Geometry check sheet. Reference: the model listing, model coordinates, mm. Give positions to 0.01 mm unless a question says otherwise; leave off trailing zeros. Write each loop counter-clockwise with the first axis right and the second up, starting at its lowest first coordinate (ties: lowest second). Pieces come first, ordered by that corner, then holes. Notation, with made-up numbers: M -9.5,-12.5 L 30.5,-12.5 A22 ccw 30.5,23.5 Z; hole C 86,77.5 d6. An arc over 180 degrees is marked long. One line per item, written item: value. Start each with the question number.
1. Cross-section at A-A on x = 38.6. Record the cut outline in (y, z), then the cut area to 3 significant figures.
2. Scan lines: line 1 (X direction, y = -7, z = 0); line 2 (Y direction, x = 5, z = 7); line 3 (Y direction, x = 146.5, z = 0.5). Record each from-to range of solid material in increasing order.
3. Gauge pin test, flat end, axial feed: pin 1 (2.5 mm diameter, centred on x = 170, y = 0, fed in from -Z). Record the tip position at first contact, or that the pin passes through.
4. Cross-section at B-B on x = 135. Record the cut outline in (y, z).
from build123d import *

# Parameters (mm, degrees)
SKETCH_1_W          = 15
SKETCH_1_H          = 15
SKETCH_1_W_2        = 13
SKETCH_1_H_2        = 13
EXTRUDE_1_DEPTH     = 185
SKETCH_2_R          = 1.45
CUT_EXTRUDE_1_DEPTH = 186.758579883
SKETCH_3_R          = 1.6
SKETCH_3_R_2        = 1.45
CUT_EXTRUDE_2_DEPTH = 186.758579883


with BuildPart() as part:
    # 草图1 → 凸台-拉伸1 (new body)
    with BuildSketch(Plane(origin=(0, 0, 0), x_dir=(0, 0, -1), z_dir=(1, 0, 0))):
        Rectangle(SKETCH_1_W, SKETCH_1_H)
        Rectangle(SKETCH_1_W_2, SKETCH_1_H_2, mode=Mode.SUBTRACT)
    extrude(amount=EXTRUDE_1_DEPTH)

    # 草图2 → 切除-拉伸1 (cut, through all)
    with BuildSketch(Plane.XY.offset(7.5)):
        with Locations((180, 0)):
            Circle(SKETCH_2_R)
        with Locations((170, 0)):
            Circle(SKETCH_2_R)
        with Locations((5, 0)):
            Circle(SKETCH_2_R)
        with Locations((15, 0)):
            Circle(SKETCH_2_R)
    extrude(amount=-CUT_EXTRUDE_1_DEPTH, mode=Mode.SUBTRACT)

    # 草图3 → 切除-拉伸2 (cut, through all)
    with BuildSketch(Plane(origin=(0, 7.5, 0), x_dir=(1, 0, 0), z_dir=(0, 1, 0))):
        with Locations(Location((38.6, 0, 0), (0, 0, 270))):
            Circle(SKETCH_3_R)
        with Locations(Location((18.6, 0, 0), (0, 0, 270))):
            Circle(SKETCH_3_R)
        with Locations(Location((53.6, 0, 0), (0, 0, 270))):
            Circle(SKETCH_3_R_2)
        with Locations(Location((58.6, 0, 0), (0, 0, 270))):
            Circle(SKETCH_3_R_2)
        with Locations(Location((73.6, 0, 0), (0, 0, 270))):
            Circle(SKETCH_3_R_2)
    extrude(amount=-CUT_EXTRUDE_2_DEPTH, mode=Mode.SUBTRACT)


solid = part.part
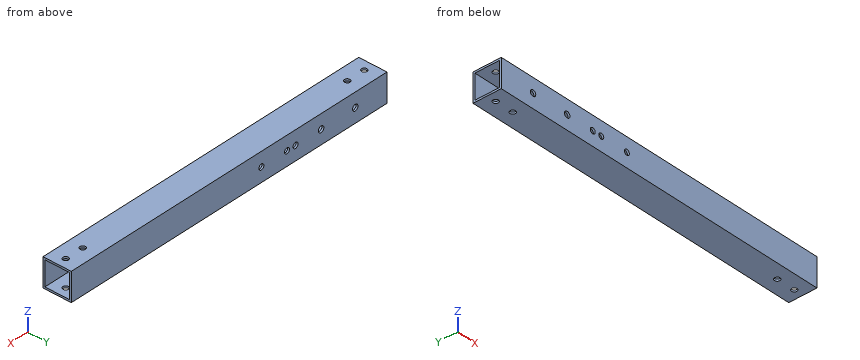
Report:
1. outline: M -7.5,-7.5 L 7.5,-7.5 L 7.5,-1.6 L 6.5,-1.6 L 6.5,-6.5 L -6.5,-6.5 L -6.5,-1.6 L -7.5,-1.6 Z; M -7.5,1.6 L -6.5,1.6 L -6.5,6.5 L 6.5,6.5 L 6.5,1.6 L 7.5,1.6 L 7.5,7.5 L -7.5,7.5 Z
1. area: 49.6 mm^2
2. line 1: x = 0 to 17, 20.2 to 37, 40.2 to 52.15, 55.05 to 57.15, 60.05 to 72.15, 75.05 to 185
2. line 2: y = -7.5 to -1.45, 1.45 to 7.5
2. line 3: y = -7.5 to -6.5, 6.5 to 7.5
3. pin 1: passes through
4. outline: M -7.5,-7.5 L 7.5,-7.5 L 7.5,7.5 L -7.5,7.5 Z; hole M -6.5,-6.5 L 6.5,-6.5 L 6.5,6.5 L -6.5,6.5 Z
